Could you check a few things on this drawing? It's one solid part, dimensions in mm from its lowest x, y, z. A direction names the side the tool comes from. Give positions to 0.01 mm unless a question says otherwise; leave off trailing zeros. Loops run counter-clockwise (first coordinate to the right, second up) from the corner with the lowest first, then second, coordinate; pieces in that order, holes last.
1. Imagine slicing it at B-B (z = 1.5). List the corners of the cut face in (x, y) for me.
2. Imagine slicing it at C-C (y = 6.5). List the corners of the cut face in (x, z) for me, plus the area to 3 significant figures.
3. For the marked faces 1 and 2, which set-ups out of +Z, -Z, +X, -X, +Y, -Y let a thin tool reach every point of the face, with its end or its side?
4. I need wall thicknesses on line 1 along Y through (x, z) = (1.35, 2.8); line 2 along X through (y, z) = (4.5, 1.5); line 3 along Y through (x, z) = (2.35, 1.7). Which ranges of each line are inside material? Lowest first, please.
5. Imagine slicing it at A-A (x = 1.5). List the corners of the cut face in (y, z) for me.
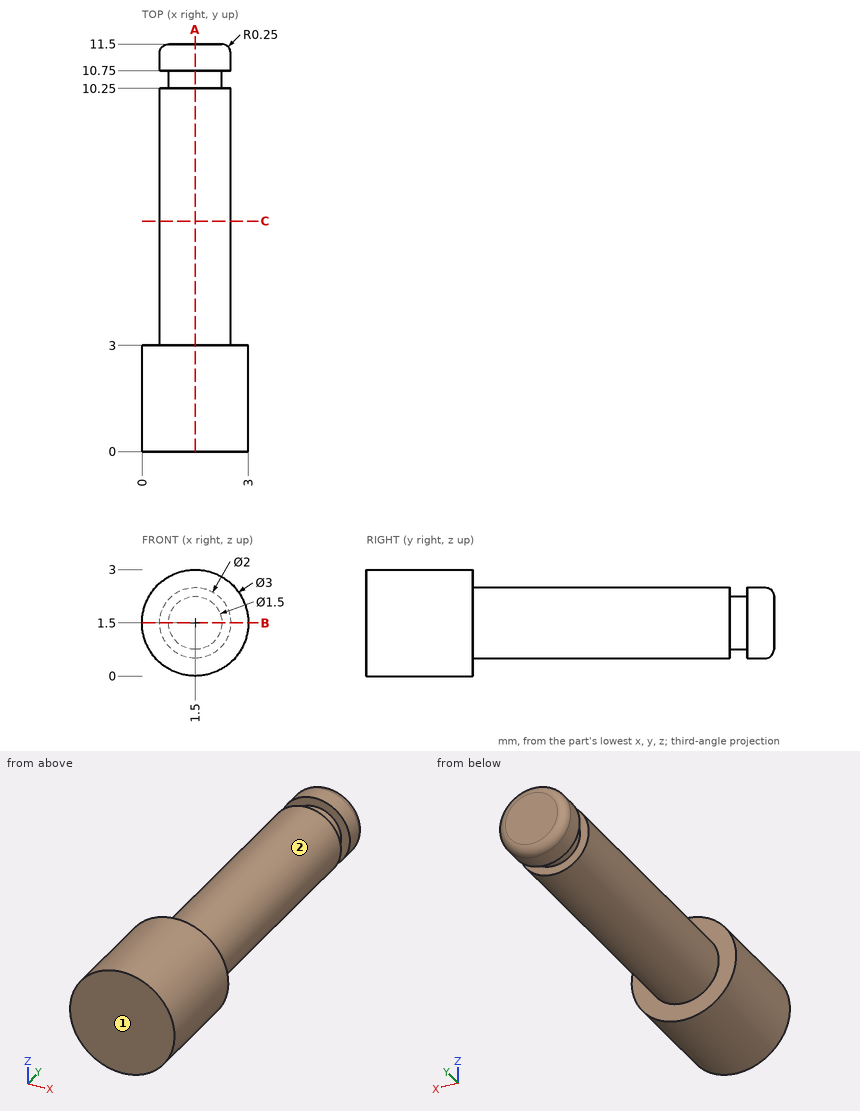
Derived:
1. outline: (0, 0) - (3, 0) - (3, 3) - (2.5, 3) - (2.5, 10.25) - (2.25, 10.25) - (2.25, 10.75) - (2.5, 10.75) - (2.5, 11.25) arc R0.25 ccw to (2.25, 11.5) - (0.75, 11.5) arc R0.25 ccw to (0.5, 11.25) - (0.5, 10.75) - (0.75, 10.75) - (0.75, 10.25) - (0.5, 10.25) - (0.5, 3) - (0, 3) - close
2. outline: circle Ø2 at (1.5, 1.5)
2. area: 3.14 mm2
3. face 1: +Z, -Z, +X, -X, -Y
3. face 2: +Y
4. line 1: y = 0 to 3
4. line 2: x = 0.5 to 2.5
4. line 3: y = 0 to 10.25, 10.75 to 11.47
5. outline: (0, 0) - (3, 0) - (3, 0.5) - (10.25, 0.5) - (10.25, 0.75) - (10.75, 0.75) - (10.75, 0.5) - (11.25, 0.5) arc R0.25 ccw to (11.5, 0.75) - (11.5, 2.25) arc R0.25 ccw to (11.25, 2.5) - (10.75, 2.5) - (10.75, 2.25) - (10.25, 2.25) - (10.25, 2.5) - (3, 2.5) - (3, 3) - (0, 3) - close
